Geometry: final body of the model. Coordinates: model frame, mm. A direction names the side the tool comes from. Coordinates: 2 decimals unless noted, no trailing zeros. Loops run counter-clockwise (first coordinate to the right, second up) from the corner with the lowest first, then second, coordinate; pieces in that order, holes last. Notation, with made-up numbers: (-26.75, -29.5) -> (7.25, -29.5) arc R11 cw to (7.25, -8.5) -> close; hole circle Ø9 at (0.25, 10.5). An arc over 180 degrees is marked (long way). One line per item, written item: value. Start each with the question number.
Item 1: Section query C-C on y = 6. Return loops of the section in (x, z).
Item 2: Section query B-B on x = 0. Return loops of the section in (y, z), then the cut area to 3 significant figures.
Item 3: Mould query, pull axis Y, two halves, no side actions, for faces 4 (the flat face through (-12.7, 30, 253)), 5 (the flat face through (8, -69.85, 253)), 6 (the flat face through (29, -52.86, 253)), 7 (the flat face through (2, 19.388, 253)). Classes: +Y half, -Y half, draft (parallel to the pull), parting line (faces both ways), or undercut.
Item 4: Contact query for flat-ended pins moving along their axis: pin 1 Ø5 at (x, z) = (25, 351) entering from +Y; pin 2 Ø5 at (y, z) = (22.5, 237) entering from +X; pin 3 Ø7 at (x, z) = (2, 280) entering from +Y. Output: stop coordinate, or through.
Item 5: Section query D-D on y = -15.5. Return loops of the section in (x, z).
Item 6: Set-up query: faces 1 (the flat face through (19.388, -6, 253)), 2 (the flat face through (38.1, -61, 253)), 3 (the flat face through (29, -44.922, 253)). Return all of +Z, -Z, +X, -X, +Y, -Y with unobstructed straight access to the full face (end or side cutting, diameter ignored); none if empty.
Item 7: Ray query, probe 1 along Y at (x, z) = (0, 252.5); probe 2 along Y at (x, z) = (32, 248); probe 3 along X at (y, z) = (-20, 465). Return the intervals inside material, ascending. Write a range as from..to.
from build123d import *

# Parameters (mm, degrees)
SKETCH1_R           = 11.1125
BOSS_EXTRUDE1_DEPTH = 513.461
SKETCH2_W           = 20.65782
SKETCH2_H           = 2.54
CUT_EXTRUDE1_DEPTH  = 2.54


with BuildPart() as part:
    # Sketch1 → Boss-Extrude1 (new body)
    with BuildSketch(Plane.XY):
        with BuildLine():
            Line((34.925, -69.85), (-19.05, -69.85))
            ThreePointArc((-19.05, -69.85), (-23.540128061, -67.990128061), (-25.4, -63.5))
            Line((-25.4, -63.5), (-25.4, 36.297819962))
            ThreePointArc((-25.4, 36.297819962), (-23.726115254, 40.338935216), (-19.685, 42.012819962))
            Line((-19.685, 42.012819962), (-18.415, 42.012819962))
            ThreePointArc((-18.415, 42.012819962), (-14.373884746, 40.338935216), (-12.7, 36.297819962))
            Line((-12.7, 36.297819962), (-12.7, 22.56282))
            ThreePointArc((-12.7, 22.56282), (-11.77006403, 20.31775597), (-9.525, 19.38782))
            Line((-9.525, 19.38782), (13.03782, 19.38782))
            ThreePointArc((13.03782, 19.38782), (17.527948061, 17.527948061), (19.38782, 13.03782))
            Line((19.38782, 13.03782), (19.38782, -25.872179904))
            ThreePointArc((19.38782, -25.872179904), (20.31775597, -28.117243934), (22.56282, -29.047179904))
            Line((22.56282, -29.047179904), (34.925, -29.047179904))
            ThreePointArc((34.925, -29.047179904), (37.17006403, -29.977115874), (38.1, -32.222179904))
            Line((38.1, -32.222179904), (38.1, -41.747179904))
            ThreePointArc((38.1, -41.747179904), (37.17006403, -43.992243934), (34.925, -44.922179904))
            Line((34.925, -44.922179904), (22.56282, -44.922179904))
            ThreePointArc((22.56282, -44.922179904), (20.31775597, -45.852115874), (19.38782, -48.097179904))
            Line((19.38782, -48.097179904), (19.38782, -49.684679904))
            ThreePointArc((19.38782, -49.684679904), (20.31775597, -51.929743934), (22.56282, -52.859679904))
            Line((22.56282, -52.859679904), (34.925, -52.859679904))
            ThreePointArc((34.925, -52.859679904), (37.17006403, -53.789615874), (38.1, -56.034679904))
            Line((38.1, -56.034679904), (38.1, -66.675))
            ThreePointArc((38.1, -66.675), (37.17006403, -68.92006403), (34.925, -69.85))
        make_face()
        Circle(SKETCH1_R, mode=Mode.SUBTRACT)
    extrude(amount=BOSS_EXTRUDE1_DEPTH)

    # Sketch2 → Cut-Extrude1 (cut)
    with BuildSketch(Plane.XY.offset(513.461)):
        with Locations((9.05891, 0)):
            Rectangle(SKETCH2_W, SKETCH2_H)
    extrude(amount=-CUT_EXTRUDE1_DEPTH, mode=Mode.SUBTRACT)


solid = part.part
Reply:
1. outline: (-25.4, 0) -> (-9.35, 0) -> (-9.35, 513.46) -> (-25.4, 513.46) -> close; (9.35, 0) -> (19.39, 0) -> (19.39, 513.46) -> (9.35, 513.46) -> close
2. outline: (-69.85, 0) -> (-11.11, 0) -> (-11.11, 513.46) -> (-69.85, 513.46) -> close; (11.11, 0) -> (19.39, 0) -> (19.39, 513.46) -> (11.11, 513.46) -> close
2. area: 34,400 mm²
3. face 4: draft
3. face 5: -Y half
3. face 6: undercut
3. face 7: +Y half
4. pin 1: stops at y = -29.05
4. pin 2: stops at x = -11.4
4. pin 3: stops at y = 19.39
5. outline: (-25.4, 0) -> (19.39, 0) -> (19.39, 513.46) -> (-25.4, 513.46) -> close
6. face 1: +Z, -Z, +X, +Y
6. face 2: +Z, -Z, +X, +Y, -Y
6. face 3: +Z, -Z, +X
7. probe 1: y = -69.85..-11.11, 11.11..19.39
7. probe 2: y = -69.85..-52.86, -44.92..-29.05
7. probe 3: x = -25.4..19.39
